```python
from build123d import *

# Parameters (mm, degrees)
SKETCH1_W           = 17
SKETCH1_H           = 17
SKETCH1_R           = 1.5
BOSS_EXTRUDE1_DEPTH = 1
SKETCH2_W           = 14.5
SKETCH2_H           = 7.2
BOSS_EXTRUDE2_DEPTH = 14
SKETCH3_W           = 12.5
SKETCH3_H           = 5.2
CUT_EXTRUDE1_DEPTH  = 10


with BuildPart() as part:
    # Sketch1 → Boss-Extrude1 (new body)
    with BuildSketch(Plane(origin=(0, 0, 0), x_dir=(1, 0, 0), z_dir=(0, 1, 0))):
        with Locations((-8.5, 8.5)):
            Rectangle(SKETCH1_W, SKETCH1_H)
        with Locations(Location((-6, 14.5, 0), (0, 0, 270))):
            Circle(SKETCH1_R, mode=Mode.SUBTRACT)
        with Locations(Location((-6, 2.5, 0), (0, 0, 270))):
            Circle(SKETCH1_R, mode=Mode.SUBTRACT)
    extrude(amount=BOSS_EXTRUDE1_DEPTH)

    # Sketch2 → Boss-Extrude2 (add)
    with BuildSketch(Plane.ZY.offset(25)):
        with Locations((-8.5, 4.6)):
            Rectangle(SKETCH2_W, SKETCH2_H)
    extrude(amount=-BOSS_EXTRUDE2_DEPTH)

    # Sketch3 → Cut-Extrude1 (cut)
    with BuildSketch(Plane.ZY.offset(25)):
        with Locations((-8.5, 4.6)):
            Rectangle(SKETCH3_W, SKETCH3_H)
    extrude(amount=-CUT_EXTRUDE1_DEPTH, mode=Mode.SUBTRACT)


solid = part.part
```
Input: part model. Units: mm. Frame: model coordinates. A direction names the side the tool comes from. Give positions to 0.01 mm unless a question says otherwise; leave off trailing zeros. Write each loop counter-clockwise with the first axis right and the second up, starting at its lowest first coordinate (ties: lowest second). Pieces come first, ordered by that corner, then holes. Notation, with made-up numbers: (-18.5, 72.5) - (0.5, 72.5) arc R18 ccw to (0.5, 103.5) - close; hole circle Ø9 at (60.5, 81). An arc over 180 degrees is marked (long way). Write item = value, one per line. Start each with the question number.
1) Cut plane D-D (z = -5). Return loops of the section in (x, y), and give its area (3 significant figures).
2) Cut plane A-A (x = -6). Return loops of the section in (y, z).
3) Cut plane B-B (x = -18). Return loops of the section in (y, z).
4) Draft query along X for faces 6 (the face through (-5.93, 0.49, -16)), 7 (the face through (-17, 0.5, -8.4)), 8 (the face through (-11, 5, -9)). Return one class per face: pulls with the +X half, pulls with the -X half, needs draft (parallel to the pull), parting line crosses it, or undercut.
5) Pin query (flat end, axial travel): pin 1 (8 mm diameter, centred on x = -22.5, z = -6.5, fed in from -Y); pin 2 (4 mm diameter, centred on x = -6, z = -2.5, fed in from +Y); pin 3 (0.8 mm diameter, centred on y = 0.5, z = -10.5, fed in from -X). Return the tip coordinate at first contact, or that it passes through.
6) Reachability of faces 1 (the face through (0, 0.5, -8.4)), 2 (the face through (-18, 5, -1.25)), 3 (the face through (-20, 5, -2.25)), 4 (the face through (-9, 0, -9)), 5 (the face through (-21, 1, -9)) from +Z, -Z, +X, -X, +Y, -Y: full face, straight path, thin tool, end or side. Return the list, or none.
7) Material intervals for L1, parallel to Z at x = -16.5, y = 3.5; L2, parallel to X at y = 0.2, z = -14.5; L3, parallel to Y at x = -22, z = -8.5, sorted ascending. Write a range as [from, to].
8) Cut plane C-C (y = 2.5). Return loops of the section in (x, z), and give its area (3 significant figures).
Answers follow:
q1.outline = (-25, 1) - (-17, 1) - (-17, 0) - (0, 0) - (0, 1) - (-11, 1) - (-11, 8.2) - (-25, 8.2) - (-25, 7.2) - (-15, 7.2) - (-15, 2) - (-25, 2) - close
q1.area = 65.8 mm^2
q2.outline = (0, -17) - (1, -17) - (1, -16) - (0, -16) - close; (0, -13) - (1, -13) - (1, -4) - (0, -4) - close; (0, -1) - (1, -1) - (1, 0) - (0, 0) - close
q3.outline = (1, -15.75) - (8.2, -15.75) - (8.2, -1.25) - (1, -1.25) - close; hole (2, -14.75) - (7.2, -14.75) - (7.2, -2.25) - (2, -2.25) - close
q4.face_6 = undercut
q4.face_7 = pulls with the -X half
q4.face_8 = pulls with the +X half
q5.pin_1 = 1
q5.pin_2 = 1
q5.pin_3 = -17
q6.face_1 = +Z, -Z, +X, +Y, -Y
q6.face_2 = +Z, +X, -X, +Y
q6.face_3 = -X
q6.face_4 = +Z, -Z, +X, -X, -Y
q6.face_5 = +Z, -Z, -X, -Y
q7.L1 = [-15.75, -14.75], [-2.25, -1.25]
q7.L2 = [-17, -7.5], [-4.5, 0]
q7.L3 = [1, 2], [7.2, 8.2]
q8.outline = (-25, -15.75) - (-11, -15.75) - (-11, -1.25) - (-25, -1.25) - (-25, -2.25) - (-15, -2.25) - (-15, -14.75) - (-25, -14.75) - close
q8.area = 78.0 mm^2
